Geometry check sheet. Reference: the model listing, model coordinates, mm. A direction names the side the tool comes from. Round coordinates to 2 decimals unless told otherwise and drop trailing zeros. Order: outer loops, then holes, each group sorted by start corner. A loop starts at its lowest first (then second) coordinate and runs counter-clockwise, first axis right, second up.
(1) Draft check along X on faces 3 (the face through (1, 28.5, 0)), 4 (the face through (-0.434, 27.754, 1.952)), 5 (the face through (0, 28, 0)). Enter one of: pulls with the +X half, pulls with the -X half, needs draft (parallel to the pull), parting line crosses it, or undercut.
(2) Thickness scan on L1, parallel to Y at x = -0.05, z = -0.1; L2, parallel to Y at x = 1.55, z = 0; L3, parallel to X at y = -24, z = 0.45. Record the ranges inside material, lowest first.
(3) Set-up check for faces 1 (the face through (-1, 27.5, -1)), 2 (the face through (0, -28.5, 0)): record each of +Z, -Z, +X, -X, +Y, -Y from which the full face is reachable in a straight line by a thin tool's end or side.
(4) Gauge pin test, flat ends, axial feed: P1, Ø0.6, axis at y = 28, z = 0.5, coming from the +X side; P2, Ø1, axis at y = -21, z = -1, coming from the -X side; P3, Ø1.5, axis at y = 19.5, z = 0, coming from the +X side. Record the tip position at first contact, or that the pin passes through.
(5) Cross-section at B-B on y = 19.5. Enter the section's corners in (x, z).
(6) Cross-section at A-A on z = 0. Enter the section's corners in (x, y).
from build123d import *

# Parameters (mm, degrees)
SKETCH2_W          = 1
SKETCH2_H          = 8
CUT_EXTRUDE1_DEPTH = 0.5


with BuildPart() as part:
    # Sketch1 → Revolve1 (revolve)
    with BuildSketch(Plane.XY):
        with BuildLine():
            Line((0, -28.5), (1.25, -28.5))
            Line((1.25, -28.5), (1.25, 27.5))
            Line((1.25, 27.5), (2, 27.5))
            Line((2, 27.5), (2, 28))
            ThreePointArc((2, 28), (1.853553391, 28.353553391), (1.5, 28.5))
            Line((1.5, 28.5), (0, 28.5))
            Line((0, 28.5), (0, -28.5))
        make_face()
    revolve(axis=Axis((0, -28.5, 0), (0, 1, 0)))

    # Sketch2 → Cut-Extrude1 (cut)
    with BuildSketch(Plane(origin=(0, 28.5, 0), x_dir=(1, 0, 0), z_dir=(0, 1, 0))):
        Rectangle(SKETCH2_W, SKETCH2_H)
    extrude(amount=-CUT_EXTRUDE1_DEPTH, mode=Mode.SUBTRACT)


solid = part.part
Found:
1. face 3: needs draft
1. face 4: parting line crosses it
1. face 5: undercut
2. L1: y = -28.5 to 28
2. L2: y = 27.5 to 28.5
2. L3: x = -1.17 to 1.17
3. face 1: -Y
3. face 2: +Z, -Z, +X, -X, -Y
4. P1: stops at x = 1.99
4. P2: stops at x = -1.15
4. P3: stops at x = 1.25
5. outline: circle Ø2.5 at (0, 0)
6. outline: (-2, 27.5) - (-1.25, 27.5) - (-1.25, -28.5) - (1.25, -28.5) - (1.25, 27.5) - (2, 27.5) - (2, 28) arc R0.5 ccw to (1.5, 28.5) - (0.5, 28.5) - (0.5, 28) - (-0.5, 28) - (-0.5, 28.5) - (-1.5, 28.5) arc R0.5 ccw to (-2, 28) - close
